Autodesk Inventor part; units mm, degrees
ref_plane "YZ Plane" through (0, 0, 0) normal (1, 0, 0) x (0, 1, 0)
ref_plane "XZ Plane" through (0, 0, 0) normal (0, 1, 0) x (-1, 0, 0)
ref_plane "XY Plane" through (0, 0, 0) normal (0, 0, 1) x (1, 0, 0)
sketch "Sketch1" plane through (0, 0, 0) normal (0, 1, 0) x (-1, 0, 0)
  line L0 (0, 0) -> (15.875, 0)
  line L1 (15.875, 0) -> (15.875, -20.828)
  line L2 (15.875, -20.828) -> (0, -20.828)
  line L3 (0, -20.828) -> (0, 0)
  line L4 (17.4625, 1.5875) -> (-1.5875, 1.5875)
  line L5 (-1.5875, 1.5875) -> (-1.5875, -22.4155)
  line L6 (-1.5875, -22.4155) -> (17.4625, -22.4155)
  line L7 (17.4625, -22.4155) -> (17.4625, 1.5875)
  dimension "d0" = 20.828
  dimension "d1" = 15.875
  dimension "d2" = 1.5875
  dimension "d3" = 1.5875
  dimension "d4" = 1.5875
  dimension "d5" = 1.5875
extrude "Extrusion1" add sketch "Sketch1" along normal blind 0.7937 contours L0 L1 L2 L3
extrude "Extrusion2" add sketch "Sketch1" along normal blind 5.5563
sketch "Sketch2" plane through (0, 0.7937, 0) normal (0, 1, 0) x (1, 0, 0)
  line L0 (0, 0) -> (-15.875, 0)
  line L1 (0, 20.828) -> (-15.875, 20.828)
  line L2 (-15.875, 20.828) -> (-15.875, 0)
  line L3 (-15.875, 0) -> (0, 0)
  line L4 (0, 0) -> (0, 20.828)
  line L5 (-15.875, 0.7938) -> (0, 0.7937)
  line L6 (0, 0.7937) -> (0, 3.9688)
  line L7 (0, 3.9688) -> (-15.875, 3.9687)
  line L8 (-15.875, 3.9687) -> (-15.875, 0.7938)
  point P0 (0, 0.7937)
  dimension "d10" = 3.175
  dimension "d11" = 0.7937
extrude "Extrusion3" cut sketch "Sketch2" against normal blind 5.5563 contours L5 L2 L7 L4
sketch "Sketch3" plane through (0, 5.5563, 0) normal (0, 1, 0) x (1, 0, 0)
  line L0 (1.5875, -1.5875) -> (1.5875, 22.4155)
  line L1 (1.5875, 22.4155) -> (-17.4625, 22.4155)
  line L2 (-17.4625, 22.4155) -> (-17.4625, -1.5875)
  line L3 (-17.4625, -1.5875) -> (1.5875, -1.5875)
  line L4 (0, 0) -> (-15.875, 0)
  line L5 (-15.875, 0) -> (-15.875, 20.828)
  line L6 (-15.875, 20.828) -> (0, 20.828)
  line L7 (0, 20.828) -> (0, 0)
  line L8 (-17.0656, -1.1906) -> (1.1906, -1.1906)
  line L9 (1.1906, -1.1906) -> (1.1906, 22.0186)
  line L10 (1.1906, 22.0186) -> (-17.0656, 22.0186)
  line L11 (-17.0656, 22.0186) -> (-17.0656, -1.1906)
  line L12 (-16.2719, -0.3969) -> (0.3969, -0.3969)
  line L13 (0.3969, -0.3969) -> (0.3969, 21.2249)
  line L14 (0.3969, 21.2249) -> (-16.2719, 21.2249)
  line L15 (-16.2719, 21.2249) -> (-16.2719, -0.3969)
  dimension "d14" = 0.3969
  dimension "d15" = 0.3969
  dimension "d16" = 0.3969
  dimension "d17" = 0.3969
  dimension "d18" = 0.3969
  dimension "d19" = 0.3969
  dimension "d20" = 0.3969
  dimension "d21" = 0.3969
extrude "Extrusion4" cut sketch "Sketch3" against normal blind 0.7937 contours L11 L10 L9 L8
fillet "Fillet1" radius 0.508 4 edges at (-17.4625, 2.7781, 1.5875) (-17.4625, 2.7781, -22.4155) (1.5875, 2.7781, -22.4155) (1.5875, 2.7781, 1.5875)
properties part number "Light Sensor Box V1_3DPrint"
Source: CAD feature listing. Evaluate the final solid. Frame: model axes, mm. A direction names the side the tool comes from. Give positions to 0.01 mm unless a question says otherwise; leave off trailing zeros. Write each loop counter-clockwise with the first axis right and the second up, starting at its lowest first coordinate (ties: lowest second). Pieces come first, ordered by that corner, then holes. Notation, with made-up numbers: M 79.25,84.25 L 120.25,84.25 A11 ccw 120.25,105.25 Z; hole C -23,83 d11. An arc over 180 degrees is marked long. Return JSON: item names as keys, results as strings. Group by question number.
1) Draft query along Z for faces 1 (the face through (-8, 3, 0)), 2 (the face through (-8, 3, 1.588)), 3 (the face through (-17.462, 3, -11)), 4 (the face through (-8, 3, -22.416)). Return one class per face: released by +Z, released by -Z, zero draft, split by the parting line, or undercut.
2) First-contact query: pin 1 Ø1 at (x, z) = (-13.5, -9) entering from +Y. Flat tip, straight axial feed; report the tip coordinate or a pass-through.
3) Set-up query: faces 5 (the face through (-15.875, 3, -11)), 6 (the face through (1.588, 3, -10)). Return all of +Z, -Z, +X, -X, +Y, -Y with unobstructed straight access to the full face (end or side cutting, diameter ignored); none if empty.
4) Cut plane A-A, the plane y = 5.05. Output: boundary loops of the cut face in (x, z) (1 decimal).
5) Cut plane B-B, the plane y = 0.45. Output: boundary loops of the cut face in (x, z) (1 decimal).
6) Cut plane C-C, the plane x = -11.5. Output: boundary loops of the cut face in (y, z).
7) Ray query, L1, parallel to Z at x = -3.75, y = 5.3; L2, parallel to X at y = 1.05, z = -18 (1 decimal); L3, parallel to Z at x = -4.75, y = 4.05. Return the intervals inside material, ascending.
Data:
{
 "1": {"face 1": "undercut", "face 2": "released by +Z", "face 3": "zero draft", "face 4": "released by -Z"},
 "2": {"pin 1": "stops at y = 0.79"},
 "3": {"face 5": "+Y", "face 6": "+Z, -Z, +X, +Y, -Y"},
 "4": {"outline": "M -17.5,-21.9 A0.5 ccw -17,-22.4 L 1.1,-22.4 A0.5 ccw 1.6,-21.9 L 1.6,1.1 A0.5 ccw 1.1,1.6 L -17,1.6 A0.5 ccw -17.5,1.1 Z; M -16.3,-21.2 L 0.4,-21.2 L 0.4,0.4 L -16.3,0.4 Z; hole M -17.1,-22 L 1.2,-22 L 1.2,1.2 L -17.1,1.2 Z; hole M -15.9,-20.8 L 0,-20.8 L 0,0 L -15.9,0 Z"},
 "5": {"outline": "M -17.5,-21.9 A0.5 ccw -17,-22.4 L 1.1,-22.4 A0.5 ccw 1.6,-21.9 L 1.6,1.1 A0.5 ccw 1.1,1.6 L -17,1.6 A0.5 ccw -17.5,1.1 Z; hole M -15.9,-4 L 0,-4 L 0,-0.8 L -15.9,-0.8 Z"},
 "6": {"outline": "M 0,-22.42 L 5.56,-22.42 L 5.56,-22.02 L 4.76,-22.02 L 4.76,-21.22 L 5.56,-21.22 L 5.56,-20.83 L 0.79,-20.83 L 0.79,-3.97 L 0,-3.97 Z; M 0,-0.79 L 0.79,-0.79 L 0.79,0 L 5.56,0 L 5.56,0.4 L 4.76,0.4 L 4.76,1.19 L 5.56,1.19 L 5.56,1.59 L 0,1.59 Z"},
 "7": {"L1": "z = -22.42 to -22.02, -21.22 to -20.83, 0 to 0.4, 1.19 to 1.59", "L2": "x = -17.5 to -15.9, 0 to 1.6", "L3": "z = -22.42 to -20.83, 0 to 1.59"}
}
